The listing builds one solid part. Answer for the finished solid, in the listing's coordinates (mm). Round coordinates to 2 decimals unless told otherwise and drop trailing zeros. Write each loop counter-clockwise with the first axis right and the second up, starting at its lowest first coordinate (ties: lowest second). Pieces come first, ordered by that corner, then holes.
Autodesk Inventor part; units mm, degrees
ref_plane "YZ Plane" through (0, 0, 0) normal (1, 0, 0) x (0, 1, 0)
ref_plane "XZ Plane" through (0, 0, 0) normal (0, 1, 0) x (-1, 0, 0)
ref_plane "XY Plane" through (0, 0, 0) normal (0, 0, 1) x (1, 0, 0)
sketch "Servo Hole" plane through (0, 0, 0) normal (0, 0, 1) x (1, 0, 0)
  line L0 (-67.0819, 53.6212) -> (-54.4839, 53.6212) construction
  line L1 (-54.4839, 53.6212) -> (-54.4839, 48.7062) construction
  line L2 (-54.4839, 21.2612) -> (-67.0819, 21.2612) construction
  circle A0 centre (-60.7829, 51.4432) radius 1.048
  line L3 (-67.0819, 48.7062) -> (-54.4839, 48.7062)
  line L4 (-67.0819, 26.1762) -> (-54.4839, 26.1762)
  line L5 (-54.4839, 37.4412) -> (-67.0819, 37.4412) construction
  line L6 (-54.4839, 48.7062) -> (-54.4839, 26.1762)
  line L7 (-54.4839, 26.1762) -> (-54.4839, 21.2612) construction
  line L8 (-67.0819, 48.7062) -> (-67.0819, 53.6212) construction
  line L9 (-67.0819, 26.1762) -> (-67.0819, 48.7062)
  line L10 (-67.0819, 21.2612) -> (-67.0819, 26.1762) construction
  line L11 (-60.7829, 53.6212) -> (-60.7829, 21.2612) construction
  circle A1 centre (-60.7829, 23.4392) radius 1.048
  point P0 (-60.7829, 37.4412)
  dimension "d0" = 32.36
  dimension "d2" = 2.178
  dimension "d3" = 2.096
  dimension "d4" = 22.53
  dimension "d5" = 2.096
  dimension "d6" = 2.178
sketch "Sketch1" plane through (0, 0, 0) normal (0, 1, 0) x (-1, 0, 0)
  line L0 (-42.598, 37.5) -> (42.598, 37.5)
  line L1 (42.598, 37.5) -> (42.598, -37.5)
  line L2 (42.598, -37.5) -> (-42.598, -37.5)
  line L3 (-42.598, -37.5) -> (-42.598, 37.5)
  line L4 (-42.598, 0) -> (42.598, 0) construction
  line L5 (0, 37.5) -> (0, -37.5) construction
  line L6 (-42.598, 37.5) -> (-30, 37.5) construction
  line L7 (-30, 37.5) -> (-30, 32.585) construction
  line L8 (-30, 5.14) -> (-42.598, 5.14) construction
  circle A0 centre (-36.299, 35.322) radius 1.048
  line L9 (-42.598, 32.585) -> (-30, 32.585)
  line L10 (-42.598, 10.055) -> (-30, 10.055)
  line L11 (-30, 21.32) -> (-42.598, 21.32) construction
  line L12 (-30, 32.585) -> (-30, 10.055)
  line L13 (-30, 10.055) -> (-30, 5.14) construction
  line L14 (-42.598, 32.585) -> (-42.598, 37.5) construction
  line L15 (-42.598, 10.055) -> (-42.598, 32.585)
  line L16 (-42.598, 5.14) -> (-42.598, 10.055) construction
  line L17 (-36.299, 37.5) -> (-36.299, 5.14) construction
  circle A1 centre (-36.299, 7.318) radius 1.048
  line L18 (30, 37.5) -> (42.598, 37.5) construction
  line L19 (42.598, 37.5) -> (42.598, 32.585) construction
  line L20 (42.598, 5.14) -> (30, 5.14) construction
  circle A2 centre (36.299, 35.322) radius 1.048
  line L21 (30, 32.585) -> (42.598, 32.585)
  line L22 (30, 10.055) -> (42.598, 10.055)
  line L23 (42.598, 21.32) -> (30, 21.32) construction
  line L24 (42.598, 32.585) -> (42.598, 10.055)
  line L25 (42.598, 10.055) -> (42.598, 5.14) construction
  line L26 (30, 32.585) -> (30, 37.5) construction
  line L27 (30, 10.055) -> (30, 32.585)
  line L28 (30, 5.14) -> (30, 10.055) construction
  line L29 (36.299, 37.5) -> (36.299, 5.14) construction
  circle A3 centre (36.299, 7.318) radius 1.048
  line L30 (-42.598, -5.14) -> (-30, -5.14) construction
  line L31 (-30, -5.14) -> (-30, -10.055) construction
  line L32 (-30, -37.5) -> (-42.598, -37.5) construction
  circle A4 centre (-36.299, -7.318) radius 1.048
  line L33 (-42.598, -10.055) -> (-30, -10.055)
  line L34 (-42.598, -32.585) -> (-30, -32.585)
  line L35 (-30, -21.32) -> (-42.598, -21.32) construction
  line L36 (-30, -10.055) -> (-30, -32.585)
  line L37 (-30, -32.585) -> (-30, -37.5) construction
  line L38 (-42.598, -10.055) -> (-42.598, -5.14) construction
  line L39 (-42.598, -32.585) -> (-42.598, -10.055)
  line L40 (-42.598, -37.5) -> (-42.598, -32.585) construction
  line L41 (-36.299, -5.14) -> (-36.299, -37.5) construction
  circle A5 centre (-36.299, -35.322) radius 1.048
  line L42 (30, -5.14) -> (42.598, -5.14) construction
  line L43 (42.598, -5.14) -> (42.598, -10.055) construction
  line L44 (42.598, -37.5) -> (30, -37.5) construction
  circle A6 centre (36.299, -7.318) radius 1.048
  line L45 (30, -10.055) -> (42.598, -10.055)
  line L46 (30, -32.585) -> (42.598, -32.585)
  line L47 (42.598, -21.32) -> (30, -21.32) construction
  line L48 (42.598, -10.055) -> (42.598, -32.585)
  line L49 (42.598, -32.585) -> (42.598, -37.5) construction
  line L50 (30, -10.055) -> (30, -5.14) construction
  line L51 (30, -32.585) -> (30, -10.055)
  line L52 (30, -37.5) -> (30, -32.585) construction
  line L53 (36.299, -5.14) -> (36.299, -37.5) construction
  circle A7 centre (36.299, -35.322) radius 1.048
  point P0 (0, 0)
  point P1 (0, 0)
  dimension "d12" = 60
  dimension "d8" = 85.196
  dimension "d9" = 75
extrude "Extrusion1" add sketch "Sketch1" along normal blind 3 contours L0 L1 L21 L27 L22 L45 L51 L46 L2 L3 L34 L36 L33 L10 L12 L9
sketch "Sketch2" plane through (0, 3, 0) normal (0, 1, 0) x (1, 0, 0)
  line L0 (-42.598, 10.055) -> (-42.598, -10.055)
  line L1 (-42.598, -37.5) -> (42.598, -37.5)
  line L2 (42.598, -10.055) -> (42.598, 10.055)
  line L3 (42.598, 37.5) -> (-42.598, 37.5)
  line L4 (26.67, -34.29) -> (-26.67, -34.29)
  line L5 (-26.67, -34.29) -> (-26.67, 34.29)
  line L6 (-26.67, 34.29) -> (26.67, 34.29)
  line L7 (26.67, 34.29) -> (26.67, -34.29)
  circle A0 centre (-24.13, 20.32) radius 1.5
  circle A1 centre (-19.05, -31.75) radius 1.5
  circle A2 centre (24.13, 19.05) radius 1.5
  line L8 (0, 37.5) -> (0, -37.5) construction
  line L9 (42.598, 0) -> (-42.598, 0) construction
  circle A3 centre (8.89, -31.75) radius 1.5
  point P0 (0, 0)
  dimension "d18" = 3
  dimension "d19" = 2.54
  dimension "d20" = 13.97
  dimension "d21" = 53.34
  dimension "d22" = 68.58
  dimension "d23" = 3
  dimension "d24" = 7.62
  dimension "d25" = 2.54
  dimension "d28" = 3
  dimension "d29" = 2.54
  dimension "d30" = 15.24
  dimension "d31" = 3
  dimension "d32" = 27.94
hole "Hole1" at (-24.13, 3, -20.32) at (24.13, 3, -19.05) at (8.89, 3, 31.75) at (-19.05, 3, 31.75) direction (0, -1, 0) diameter 2.459 end through all
properties part number "Base"
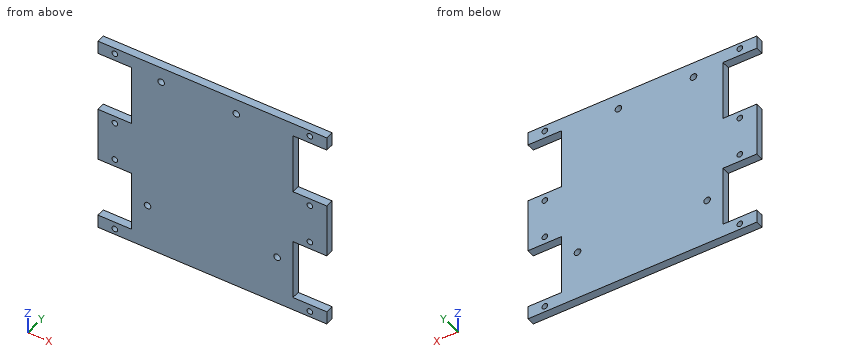
1. Section C-C on y = 0.65 is taken. Give the number of separate pieces and of enclosed holes in the cut face, plus the area to 3 significant figures.
Geometry says:
separate pieces: 1
enclosed holes: 12
area: 5,210 mm2
2. Given pin 1 (1.5 mm diameter, centred on y = 1, z = 25.5, fed in from -X), flat-ended and moving along its own axis, determine where the tip first touches the part or whether it passes through.
Geometry says:
pin 1: stops at x = -30
3. Section D-D on z = -12.5 is taken. Determine the outline of the cut face in (x, y), plus the area to 3 significant figures.
Geometry says:
outline: (-30, 0) - (30, 0) - (30, 3) - (-30, 3) - close
area: 180 mm2
4. Straight lines are drawn through the part: line 1 along X through (y, z) = (0.5, 7.5); line 2 along Z through (x, y) = (-38, 2.75) (3 decimals); line 3 along X through (y, z) = (1.65, -20.32). For each, find the intervals that lie inside material, in ascending order.
Geometry says:
line 1: x = -42.6 to -37.33, -35.27 to 35.27, 37.33 to 42.6
line 2: z = -37.5 to -32.585, -10.055 to 10.055, 32.585 to 37.5
line 3: x = -30 to -25.36, -22.9 to 30
5. Section A-A on x = -24.13 is taken. Determine the outline of the cut face in (y, z), plus the area to 3 significant figures.
Geometry says:
outline: (0, -37.5) - (3, -37.5) - (3, -21.55) - (0, -21.55) - close; (0, -19.09) - (3, -19.09) - (3, 37.5) - (0, 37.5) - close
area: 218 mm2
6. Section B-B on x = 31.5 is taken. Determine the outline of the cut face in (y, z) (3 decimals).
Geometry says:
outline: (0, -37.5) - (3, -37.5) - (3, -32.585) - (0, -32.585) - close; (0, -10.055) - (3, -10.055) - (3, 10.055) - (0, 10.055) - close; (0, 32.585) - (3, 32.585) - (3, 37.5) - (0, 37.5) - close
